Part model, mm, in its own coordinate system. A direction names the side the tool comes from. Give positions to 0.01 mm unless a question says otherwise; leave off trailing zeros. One line per item, written item: value.
```python
from build123d import *

# Parameters (mm, degrees)
SKETCH018_R         = 75
SKETCH018_W         = 5
SKETCH018_H         = 20
PAD018_DEPTH        = 5
CUT_PLACEMENT_ANGLE = 90


with BuildPart() as revolution:
    # Sketch019 → Revolution (revolve)
    with BuildSketch(Plane.XZ):
        with BuildLine():
            Line((-75, 0), (-75, 5))
            Line((-75, 5), (-70.356236, 5))
            ThreePointArc((-70.356236, 5), (-72.721103, 2.539923), (-75, 0))
        make_face()
    revolve(axis=Axis((0, 0, 0), (0, 0, 1)))


with BuildPart() as bowlsupport:
    # Sketch018 → Pad018 (new body)
    with BuildSketch(Plane.XY):
        Circle(SKETCH018_R)
        with Locations((-38.5, 0)):
            Rectangle(SKETCH018_W, SKETCH018_H, mode=Mode.SUBTRACT)
        with Locations((38.5, 0)):
            Rectangle(SKETCH018_W, SKETCH018_H, mode=Mode.SUBTRACT)
    extrude(amount=PAD018_DEPTH)

    # Cut: cut Revolution
    add(revolution.part, mode=Mode.SUBTRACT)


with BuildPart() as bowlsupport_1:
    # Cut placement: moved
    add(bowlsupport.part.moved(Location((0, 36, 160))).rotate(Axis((0, 36, 160), (0, 0, 1)), CUT_PLACEMENT_ANGLE))


solid = bowlsupport_1.part
```
1) Pin check, flat tips, straight feed: pin 1 (2.5 mm diameter, centred on y = -1.5, z = 163, fed in from +X); pin 2 (2 mm diameter, centred on y = 40, z = 162.5, fed in from -X); pin 3 (1 mm diameter, centred on x = -13, z = 163.5, fed in from +Y). Stop position of each tip, or through.
Outcome:
pin 1: stops at x = 63.34
pin 2: stops at x = -73.57
pin 3: stops at y = 107.12
2) Mould opens along X. For faces 1 (the flat face through (-1, 35, 160)), 2 (the flat face through (0, -5, 162)) say: released by +X, released by -X, zero draft, split by the parting line, or undercut.
Outcome:
face 1: zero draft
face 2: undercut
3) Which spindle directions (+Z, -Z, +X, -X, +Y, -Y) get a long thin tool onto all of the face, cutting with end or side? Do faces 3 (the flat face through (-10, 74, 162)), 4 (the flat face through (-1, 35, 165)). Say none if no direction does.
Outcome:
face 3: +Z, -Z
face 4: +Z, +X, -X, +Y, -Y
4) Drill centre lines: line 1 along Y through (x, z) = (8.5, 161.05); line 2 along Y through (x, z) = (6.5, 161.7); line 3 along X through (y, z) = (34, 163.15). Where is each one in solid material? Low to high. Write a range as from..to.
Outcome:
line 1: y = -37.59..-5, 0..72, 77..109.59
line 2: y = -37.2..-5, 0..72, 77..109.2
line 3: x = -72.12..72.12
5) Cut at A-A, the plane x = 5. Give the number of separate pieces and of enclosed holes in the cut face, then the cut area to 3 significant figures.
Outcome:
separate pieces: 3
enclosed holes: 0
area: 676 mm^2
